Read the model definition and answer for the solid it produces. Units are mm, in the model's axes. A direction names the side the tool comes from. Coordinates: 2 decimals unless noted, no trailing zeros. Order: outer loops, then holes, each group sorted by start corner. A loop starts at its lowest first (then second) coordinate and runs counter-clockwise, first axis right, second up. Notation, with made-up numbers: (-5, 21.5) -> (53, 21.5) arc R32 ccw to (53, 49.5) -> close; hole circle Ø6 at (16.5, 76). An arc over 180 degrees is marked (long way). Answer as a JSON object with one key per item and string values. Group by question number.
1) Consider L1, parallel to Y at x = 0, z = 4.7 (3 decimals); L2, parallel to Y at x = 48, z = 5.15; L3, parallel to X at y = 25, z = 2. Determine where each line is inside the solid, lowest interval first.
2) A tool of negligible diameter and unlimited length cuts with its end or side. For faces 1 (the flat face through (44, 8.5, 3)), 2 (the cylindrical face through (53.02, 2.3, 2.96)), 3 (the flat face through (43, -8.5, 3)), from which of +Z, -Z, +X, -X, +Y, -Y can it reach the whole face along a straight path? Write none if from no direction.
3) Section A-A on x = 0 is taken. Determine the outline of the cut face in (y, z) (3 decimals), and give its area (3 significant figures).
4) Section D-D on x = 41 is taken. Determine the outline of the cut face in (y, z).
5) Determine the mould class of faces 4 (the flat face through (10, 1, 6)), 5 (the cylindrical face through (-37.97, -1.55, 2.96)), 6 (the cylindrical face through (53.02, -3.2, 2.96)) for opening direction X: released by +X, released by -X, zero draft, split by the parting line, or undercut.
6) Given pin 1 (1.8 mm diameter, centred on x = 51.59, y = 2.75, fed in from +Z); pin 2 (1.5 mm diameter, centred on x = 17.5, z = 2.5, fed in from -Y), each flat-ended and moving along its own axis, determine where each tip first touches the part or whether it passes through.
7) Section C-C on y = 0 is taken. Determine the outline of the cut face in (x, z) (3 decimals).
8) Section B-B on z = 2.1 is taken. Determine the outline of the cut face in (x, y) (3 decimals).
Autodesk Inventor part; units mm, degrees
ref_plane "YZ Plane" through (0, 0, 0) normal (1, 0, 0) x (0, 1, 0)
ref_plane "XZ Plane" through (0, 0, 0) normal (0, 1, 0) x (-1, 0, 0)
ref_plane "XY Plane" through (0, 0, 0) normal (0, 0, 1) x (1, 0, 0)
sketch "スケッチ1" plane through (0, 0, 0) normal (0, 0, 1) x (1, 0, 0)
  circle A0 centre (0, 0) radius 38
  line L0 (0, 0) -> (50, 0) construction
  line L1 (0, -8.5) -> (50, -8.5)
  line L2 (50, 8.5) -> (0, 8.5)
  arc A1 (0, 8.5) -> (0, -8.5) centre (0, 0) ccw
  arc A2 (50, -8.5) -> (50, 8.5) centre (50, 0) ccw
  line L3 (46.8246, 0) -> (51.5877, 2.75) construction
  line L4 (51.5877, 2.75) -> (51.5877, -2.75) construction
  line L5 (51.5877, -2.75) -> (46.8246, 0) construction
  circle A3 centre (51.5877, 2.75) radius 1.5
  circle A4 centre (46.8246, 0) radius 1.5
  circle A5 centre (51.5877, -2.75) radius 1.5
  circle A6 centre (0, 0) radius 2.995
  point P0 (25, 0)
  dimension "d0" = 76
  dimension "d2" = 50
  dimension "d3" = 17
  dimension "d4" = 3
  dimension "d5" = 3
  dimension "d6" = 3
  dimension "d7" = 5.5
  dimension "d8" = 5.99
extrude "押し出し1" add sketch "スケッチ1" along normal blind 6
properties part number "アーム最終段円盤" material "アルミニウム 7075"
Worked answers:
{
 "1": {"L1": "y = -38 to -2.995, 2.995 to 38", "L2": "y = -8.5 to -0.93, 0.93 to 8.5", "L3": "x = -28.62 to 28.62"},
 "2": {"face 1": "+Z, -Z, +X, +Y", "face 2": "+Z, -Z", "face 3": "+Z, -Z, +X, -Y"},
 "3": {"outline": "(-38, 0) -> (-2.995, 0) -> (-2.995, 6) -> (-38, 6) -> close; (2.995, 0) -> (38, 0) -> (38, 6) -> (2.995, 6) -> close", "area": "420 mm²"},
 "4": {"outline": "(-8.5, 0) -> (8.5, 0) -> (8.5, 6) -> (-8.5, 6) -> close"},
 "5": {"face 4": "zero draft", "face 5": "split by the parting line", "face 6": "undercut"},
 "6": {"pin 1": "passes through", "pin 2": "stops at y = -34.11"},
 "7": {"outline": "(-38, 0) -> (-2.995, 0) -> (-2.995, 6) -> (-38, 6) -> close; (2.995, 0) -> (45.325, 0) -> (45.325, 6) -> (2.995, 6) -> close; (48.325, 0) -> (58.5, 0) -> (58.5, 6) -> (48.325, 6) -> close"},
 "8": {"outline": "(37.037, -8.5) -> (50, -8.5) arc R8.5 ccw to (50, 8.5) -> (37.037, 8.5) arc R38 ccw (long way) to start; hole circle Ø5.99 at (0, 0); hole circle Ø3 at (46.825, 0); hole circle Ø3 at (51.588, -2.75); hole circle Ø3 at (51.588, 2.75)"}
}
